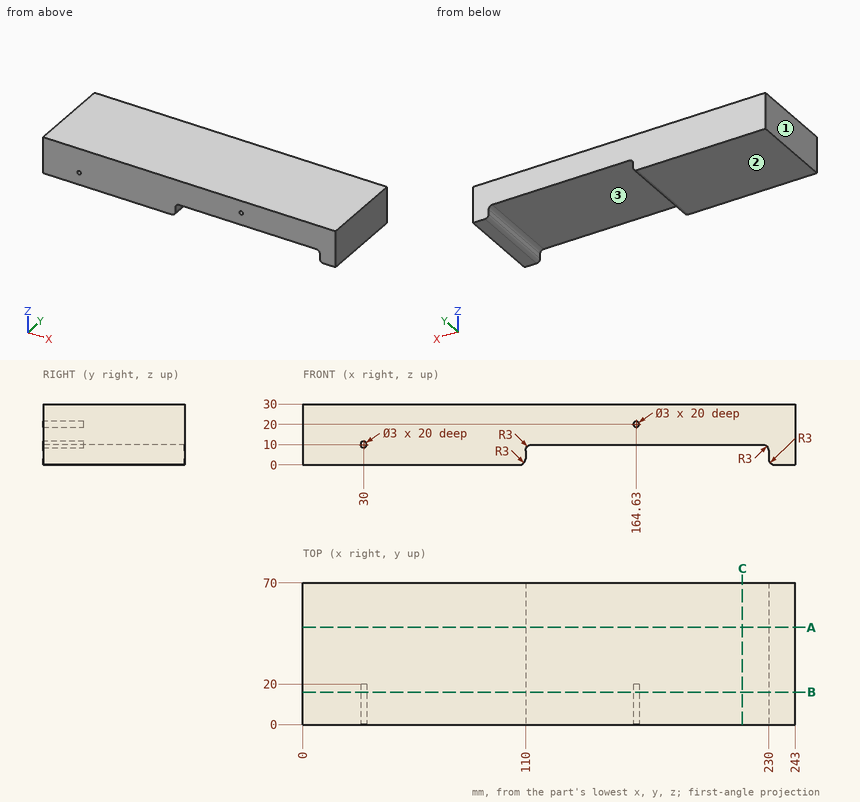
Input: dimensioned drawing with shaded views. Units: mm. Origin: part minimum x, y, z. Coordinates: 2 decimals unless noted, no trailing zeros. Order: outer loops, then holes, each group sorted by start corner. A loop starts at its lowest first (then second) coordinate and runs counter-clockwise, first axis right, second up.
Item 1: Draft query along X for the marked faces 1, 2 and 3. Return one class per face: released by +X, released by -X, zero draft, split by the parting line, or undercut.
Answer:
face 1: released by -X
face 2: zero draft
face 3: undercut
Item 2: Contact query for a flat-ended pin moving along its axis: P1, Ø0.9, axis at x = 30, z = 10, coming from the -Y side. Output: stop coordinate, or through.
Answer:
P1: stops at y = 20
Item 3: Section query A-A (y = 48). Output: boundary loops of the cut face in (x, z).
Answer:
outline: (0, 0) - (107, 0) arc R3 ccw to (110, 3) - (110, 7) arc R3 cw to (113, 10) - (227, 10) arc R3 cw to (230, 7) - (230, 3) arc R3 ccw to (233, 0) - (243, 0) - (243, 30) - (0, 30) - close
Item 4: Section query C-C (x = 217). Output: boundary loops of the cut face in (y, z).
Answer:
outline: (0, 10) - (70, 10) - (70, 30) - (0, 30) - close
Item 5: Section query B-B (y = 16). Output: boundary loops of the cut face in (x, z), then the cut area to 3 significant figures.
Answer:
outline: (0, 0) - (107, 0) arc R3 ccw to (110, 3) - (110, 7) arc R3 cw to (113, 10) - (227, 10) arc R3 cw to (230, 7) - (230, 3) arc R3 ccw to (233, 0) - (243, 0) - (243, 30) - (0, 30) - close; hole circle Ø3 at (30, 10); hole circle Ø3 at (164.63, 20)
area: 6,080 mm2
Item 6: Material intervals for line 1 along X through (y, z) = (11.5, 20); line 2 along Z through (x, y) = (164.63, 10.5); line 3 along Z through (x, y) = (30, 15.75), sorted ascending.
Answer:
line 1: x = 0 to 163.13, 166.13 to 243
line 2: z = 10 to 18.5, 21.5 to 30
line 3: z = 0 to 8.5, 11.5 to 30
